from build123d import *

# Parameters (mm, degrees)
SKETCH2_W             = 120.65
SKETCH2_H             = 25.4
BOSS_EXTRUDE2_DEPTH   = 228.6
F_4_40_TAPPED_HOLE2_D = 2.2606
SKETCH3_W             = 13.65
SKETCH3_H             = 222.560167774
CUT_EXTRUDE2_DEPTH    = 228.6
SKETCH9_W             = 216.560167774
SKETCH9_H             = 13.4
CUT_EXTRUDE3_DEPTH    = 228.6
SKETCH12_W            = 16.47911479
SKETCH12_H            = 16.039471942
BOSS_EXTRUDE4_DEPTH   = 15.81
SKETCH13_R            = 4.064
CUT_EXTRUDE4_DEPTH    = 21.81


with BuildPart() as part:
    # Sketch2 → Boss-Extrude2 (new body)
    with BuildSketch(Plane.XY):
        Rectangle(SKETCH2_W, SKETCH2_H)
    extrude(amount=BOSS_EXTRUDE2_DEPTH)

    # #4-40 Tapped Hole2 (through all)
    with Locations(Plane.XY.offset(228.6)):
        with Locations((-55.626, 8.5698965), (-55.626, -8.5698965), (55.626, 8.5698965), (55.626, -8.5698965)):
            Hole(F_4_40_TAPPED_HOLE2_D / 2)

    # Sketch3 → Cut-Extrude2 (cut)
    with BuildSketch(Plane.XZ.offset(12.7)):
        Polygon((-40.325, 6.039832226), (-40.325, 0), (40.325, 0), (40.325, 6.039832226), (40.325, 222.25), (-40.325, 222.25), align=None)
        with Locations((-53.5, 117.319916113)):
            Rectangle(SKETCH3_W, SKETCH3_H)
        with Locations((53.5, 117.319916113)):
            Rectangle(SKETCH3_W, SKETCH3_H)
    extrude(amount=-CUT_EXTRUDE2_DEPTH, mode=Mode.SUBTRACT)

    # Sketch9 → Cut-Extrude3 (cut)
    with BuildSketch(Plane.ZY.offset(46.675)):
        with Locations((114.319916113, 0)):
            Rectangle(SKETCH9_W, SKETCH9_H)
    extrude(amount=-CUT_EXTRUDE3_DEPTH, mode=Mode.SUBTRACT)

    # Sketch12 → Boss-Extrude4 (add)
    with BuildSketch(Plane(origin=(0, 0, 222.6), x_dir=(-1, 0, 0), z_dir=(0, 0, -1))):
        Rectangle(SKETCH12_W, SKETCH12_H)
    extrude(amount=BOSS_EXTRUDE4_DEPTH)

    # Sketch13 → Cut-Extrude4 (cut)
    with BuildSketch(Plane.ZY.offset(8.239557395)):
        with Locations((212.3276832, 0)):
            Circle(SKETCH13_R)
    extrude(amount=-CUT_EXTRUDE4_DEPTH, mode=Mode.SUBTRACT)


solid = part.part
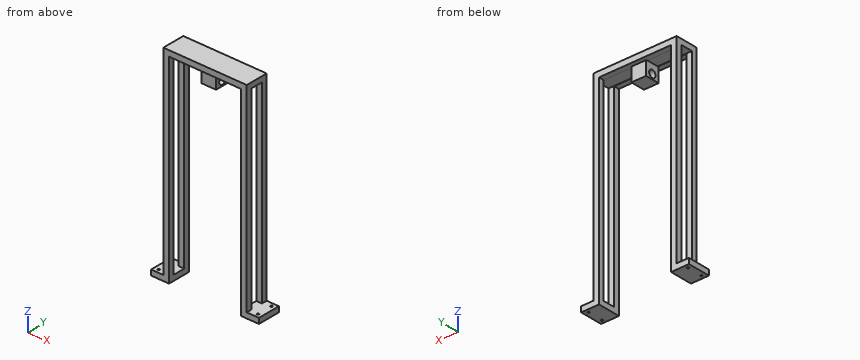
Verification items for the finished model (mm, model axes). Round coordinates to 2 decimals unless told otherwise and drop trailing zeros. Loops run counter-clockwise (first coordinate to the right, second up) from the corner with the lowest first, then second, coordinate; pieces in that order, holes last. Notation, with made-up numbers: (-0.5, -16.75) - (30.5, -16.75) arc R26 ccw to (30.5, 17.25) - close; hole circle Ø10 at (-40, -35). An arc over 180 degrees is marked (long way). Use a Markdown table: item, result. Add a question column.
1. Section check B-B, the plane z = 150. Record the boundary of the cut face in (x, y) (3 decimals), plus the area to 3 significant figures.
2. Gauge pin test, flat ends, axial feed: pin 1 (2.5 mm diameter, centred on x = 55.63, y = 8.57, fed in from +Z); pin 2 (12.5 mm diameter, centred on x = 3.5, z = 211, fed in from +Y); pin 3 (12 mm diameter, centred on y = 3.5, z = 74.5, fed in from +X) (3 decimals); pin 4 (4.5 mm diameter, centred on y = -0.5, z = 211, fed in from -X). Record the tip position at first contact, or that the pin passes through.
3. Thickness scan on probe 1 along X at (y, z) = (11.75, 215) (3 decimals); probe 2 along Z at (x, y) = (2, 0.5); probe 3 along Z at (x, y) = (44.5, 6.5). Record the ranges inside material, lowest first. Write a range as [from, to].
4. Section check A-A, the plane y = 0. Record the boundary of the cut face in (x, z) (3 decimals), plus the area to 3 significant figures.
5. Section check C-C, the plane x = -26. Record the boundary of the cut face in (y, z).
Checks:
| question | item | result |
|---|---|---|
| 1 | outline | (-46.675, -12.7) - (-40.325, -12.7) - (-40.325, -6.7) - (-46.675, -6.7) - close; (-46.675, 6.7) - (-40.325, 6.7) - (-40.325, 12.7) - (-46.675, 12.7) - close; (40.325, -12.7) - (46.675, -12.7) - (46.675, -6.7) - (40.325, -6.7) - close; (40.325, 6.7) - (46.675, 6.7) - (46.675, 12.7) - (40.325, 12.7) - close |
| 1 | area | 152 mm^2 |
| 2 | pin 1 | stops at z = 6.04 |
| 2 | pin 2 | stops at y = 8.02 |
| 2 | pin 3 | stops at x = 46.675 |
| 2 | pin 4 | passes through |
| 3 | probe 1 | x = [-46.675, -40.325], [40.325, 46.675] |
| 3 | probe 2 | z = [206.79, 208.29], [216.36, 228.6] |
| 3 | probe 3 | z = [0, 6.04], [222.6, 228.6] |
| 4 | outline | (-60.325, 0) - (-40.325, 0) - (-40.325, 6.04) - (-60.325, 6.04) - close; (-46.675, 222.6) - (-8.24, 222.6) - (-8.24, 216.392) - (8.24, 216.392) - (8.24, 222.6) - (46.675, 222.6) - (46.675, 228.6) - (-46.675, 228.6) - close; (-8.24, 206.79) - (8.24, 206.79) - (8.24, 208.264) - (-8.24, 208.264) - close; (40.325, 0) - (60.325, 0) - (60.325, 6.04) - (40.325, 6.04) - close |
| 4 | area | 928 mm^2 |
| 5 | outline | (-12.7, 222.25) - (-6.7, 222.25) - (-6.7, 222.6) - (6.7, 222.6) - (6.7, 222.25) - (12.7, 222.25) - (12.7, 228.6) - (-12.7, 228.6) - close |
